Read the model definition and answer for the solid it produces. Units are mm, in the model's axes. A direction names the side the tool comes from. Coordinates: 2 decimals unless noted, no trailing zeros. Order: outer loops, then holes, each group sorted by start corner. A loop starts at its lowest first (then second) coordinate and runs counter-clockwise, first axis right, second up. Notation, with made-up numbers: (26, 68) -> (72, 68) arc R33 cw to (72, 97) -> close; hole circle Ø6 at (-2.75, 76). An arc over 180 degrees is marked (long way). Use CSV: the item, a comma, the result in double quotes.
```python
from build123d import *

# Parameters (mm, degrees)
F0_W           = 38.1
F0_H           = 38.1
F0_R           = 6.35
F0_H_2         = 22.86
F1_DEPTH       = 6.35
F2_D           = 4.4958
F5_D           = 2.7051
F5_DEPTH       = 12.54125
F5_TIP         = 0.8126940303
F5_ON_F3_D     = 2.7051
F5_ON_F3_DEPTH = 12.54125
F5_ON_F3_TIP   = 0.8126940303


with BuildPart() as f1:
    # F0 (on Top) → F1 (new body)
    with BuildSketch(Plane.XY):
        Rectangle(F0_W, F0_H)
        Circle(F0_R, mode=Mode.SUBTRACT)
        with Locations((0, -30.48)):
            Rectangle(F0_W, F0_H_2)
        with Locations((0, -60.96)):
            Rectangle(F0_W, F0_H)
        with Locations((0, -60.96)):
            Circle(F0_R, mode=Mode.SUBTRACT)
    extrude(amount=F1_DEPTH)

    # F2 (through all)
    with Locations(Plane(origin=(0, 0, 0), x_dir=(1, 0, 0), z_dir=(0, 0, -1))):
        with Locations((-13.4747, -13.4747), (13.4747, -13.4747), (13.4747, 13.4747), (-13.4747, 13.4747), (-13.4747, 47.4853), (13.4747, 47.4853), (13.4747, 74.4347), (-13.4747, 74.4347)):
            Hole(F2_D / 2)

    # F5
    with Locations(Plane(origin=(0, 19.05, 0), x_dir=(-1, 0, 0), z_dir=(0, 1, 0))):
        with Locations((-6.91388, 3.175), (6.91388, 3.175)):
            Hole(F5_D / 2, depth=F5_DEPTH)
            with Locations((0, 0, -(F5_DEPTH + F5_TIP / 2))):  # 118° drill point
                Cone(0, F5_D / 2, F5_TIP, mode=Mode.SUBTRACT)

    # F5 on F3
    with Locations(Plane.XZ.offset(80.01)):
        with Locations((6.91388, 3.175), (-6.91388, 3.175)):
            Hole(F5_ON_F3_D / 2, depth=F5_ON_F3_DEPTH)
            with Locations((0, 0, -(F5_ON_F3_DEPTH + F5_ON_F3_TIP / 2))):  # 118° drill point
                Cone(0, F5_ON_F3_D / 2, F5_ON_F3_TIP, mode=Mode.SUBTRACT)


solid = f1.part
```
Item 1: Straight lines are drawn through the part: line 1 along Y through (x, z) = (0, 5.25); line 2 along Y through (x, z) = (-12, 3.5); line 3 along X through (y, z) = (15, 6.25). For each, find the intervals that lie inside material, in ascending order.
Return value:
line 1,"y = -80.01 to -67.31, -54.61 to -6.35, 6.35 to 19.05"
line 2,"y = -80.01 to -76.13, -72.74 to -49.18, -45.79 to -15.17, -11.78 to 11.78, 15.17 to 19.05"
line 3,"x = -19.05 to -15.13, -11.82 to 11.82, 15.13 to 19.05"
Item 2: Find section A-A, the plane y = 0. Give the vertices of the cut face in (x, z), then the cut area to 3 significant figures.
Return value:
outline,"(-19.05, 0) -> (-6.35, 0) -> (-6.35, 6.35) -> (-19.05, 6.35) -> close; (6.35, 0) -> (19.05, 0) -> (19.05, 6.35) -> (6.35, 6.35) -> close"
area,"161 mm^2"
Item 3: A tool of negligible diameter and unlimited length cuts with its end or side. For faces 5 (the cylindrical face through (-6.187, 12.692, 4.315)), 6 (the flat face through (0, -30, 0)), 7 (the cylindrical face through (6.187, -73.652, 4.315)), from which of +Z, -Z, +X, -X, +Y, -Y can it reach the whole face along a straight path? Write none if from no direction.
Return value:
face 5,"+Y"
face 6,"-Z, +X, -X, +Y, -Y"
face 7,"-Y"
Item 4: Find section C-C, the plane x = -14. Give the vertices of the cut face in (y, z), then the cut area to 3 significant figures.
Return value:
outline,"(-80.01, 0) -> (-76.62, 0) -> (-76.62, 6.35) -> (-80.01, 6.35) -> close; (-72.25, 0) -> (-49.67, 0) -> (-49.67, 6.35) -> (-72.25, 6.35) -> close; (-45.3, 0) -> (-15.66, 0) -> (-15.66, 6.35) -> (-45.3, 6.35) -> close; (-11.29, 0) -> (11.29, 0) -> (11.29, 6.35) -> (-11.29, 6.35) -> close; (15.66, 0) -> (19.05, 0) -> (19.05, 6.35) -> (15.66, 6.35) -> close"
area,"518 mm^2"
Item 5: Find section B-B, the plane x = 0. Give the vertices of the cut face in (y, z), then the cut area to 3 significant figures.
Return value:
outline,"(-80.01, 0) -> (-67.31, 0) -> (-67.31, 6.35) -> (-80.01, 6.35) -> close; (-54.61, 0) -> (-6.35, 0) -> (-6.35, 6.35) -> (-54.61, 6.35) -> close; (6.35, 0) -> (19.05, 0) -> (19.05, 6.35) -> (6.35, 6.35) -> close"
area,"468 mm^2"
Item 6: Each of these flat-tipped pins is pushed along its axis until it touches: P1, Ø4, axis at x = 13.47, y = 13.47, coming from the +Z side; P2, Ø2, axis at x = 6.91, z = 3.18, coming from the -Y side; P3, Ø2.5, axis at x = 6.91, z = 3.18, coming from the -Y side. Where does it stop, or does it pass through?
Return value:
P1,"passes through"
P2,"stops at y = -67.26"
P3,"stops at y = -67.41"
Item 7: Find section D-D, the plane x = 4.5. Give the vertices of the cut face in (y, z), then the cut area to 3 significant figures.
Return value:
outline,"(-80.01, 0) -> (-65.44, 0) -> (-65.44, 6.35) -> (-80.01, 6.35) -> close; (-56.48, 0) -> (-4.48, 0) -> (-4.48, 6.35) -> (-56.48, 6.35) -> close; (4.48, 0) -> (19.05, 0) -> (19.05, 6.35) -> (4.48, 6.35) -> close"
area,"515 mm^2"
Item 8: The mould has two halves that part along Y. Classify faces 1 (the conical face through (6.727, -66.797, 3.032)), 2 (the conical face through (7.15, 5.84, 3.19)), 3 (the cylindrical face through (11.33, 12.8, 3.22)), 4 (the flat face through (-19.05, -30, 3)): +Y half, -Y half, draft (parallel to the pull), parting line (faces both ways), or undercut.
Return value:
face 1,"-Y half"
face 2,"+Y half"
face 3,"undercut"
face 4,"draft"
